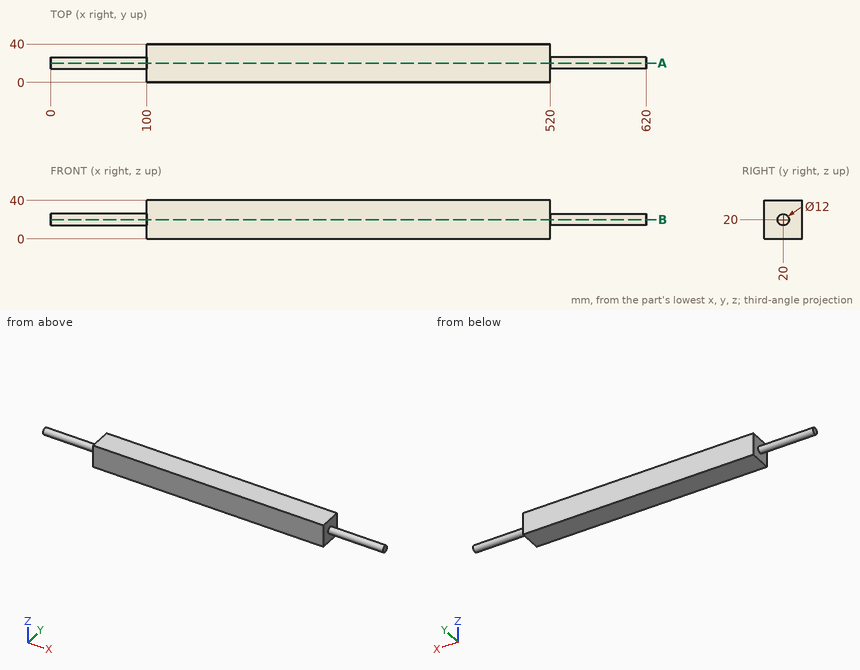
Input: dimensioned drawing with shaded views. Units: mm. Origin: part minimum x, y, z. Coordinates: 2 decimals unless noted, no trailing zeros. Order: outer loops, then holes, each group sorted by start corner. A loop starts at its lowest first (then second) coordinate and runs counter-clockwise, first axis right, second up. Notation, with made-up numbers: (-25.5, 42) -> (-12.5, 42) arc R29 cw to (-12.5, 64) -> close; hole circle Ø6 at (9.25, 21). An arc over 180 degrees is marked (long way). Answer in a Markdown table with one row per item.
Item 1: Ray query, L1, parallel to X at y = 29, z = 16.5; L2, parallel to Y at x = 27, z = 18.5; L3, parallel to Z at x = 582, y = 25.5. Return the intervals inside material, ascending.
Return value:
| item | result |
|---|---|
| L1 | x = 100 to 520 |
| L2 | y = 14.19 to 25.81 |
| L3 | z = 17.6 to 22.4 |
Item 2: Section A-A on y = 20. Output: boundary loops of the cut face in (x, z), plus the area to 3 significant figures.
Return value:
| item | result |
|---|---|
| outline | (0, 14) -> (100, 14) -> (100, 0) -> (520, 0) -> (520, 14) -> (620, 14) -> (620, 26) -> (520, 26) -> (520, 40) -> (100, 40) -> (100, 26) -> (0, 26) -> close |
| area | 19,200 mm² |
